```python
from build123d import *

# Parameters (mm, degrees)
SKETCH1_W                = 622.3
SKETCH1_H                = 38.1
BOSS_EXTRUDE1_DEPTH      = 6.35
SKETCH2_R                = 11
CUT_EXTRUDE1_DEPTH       = 1
CUT_EXTRUDE1_DEPTH_BACK  = 7.62
F_0_257_DIAMETER_HOLE2_D = 6.5278


with BuildPart() as part:
    # Sketch1 → Boss-Extrude1 (new body)
    with BuildSketch(Plane(origin=(0, 0, 0), x_dir=(1, 0, 0), z_dir=(0, 1, 0))):
        Rectangle(SKETCH1_W, SKETCH1_H)
    extrude(amount=BOSS_EXTRUDE1_DEPTH)

    # Sketch2 → Cut-Extrude1 (cut, two sides)
    with BuildSketch(Plane(origin=(0, 6.35, 0), x_dir=(1, 0, 0), z_dir=(0, 1, 0))) as cut_extrude1_sk:
        Circle(SKETCH2_R)
    extrude(amount=CUT_EXTRUDE1_DEPTH, mode=Mode.SUBTRACT)
    extrude(cut_extrude1_sk.sketch, amount=-CUT_EXTRUDE1_DEPTH_BACK, mode=Mode.SUBTRACT)

    # F (0.257) Diameter Hole2 (through all)
    with Locations(Plane(origin=(0, 6.35, 0), x_dir=(1, 0, 0), z_dir=(0, 1, 0))):
        with Locations((-279.4, 0), (-241.3, 0)):
            f_0_257_diameter_hole2 = Hole(F_0_257_DIAMETER_HOLE2_D / 2)

    # Mirror1: F (0.257) Diameter Hole2 across plane
    add(f_0_257_diameter_hole2.mirror(Plane(origin=(0, 0, 0), x_dir=(0, 0, 1), z_dir=(1, 0, 0))), mode=Mode.SUBTRACT)


solid = part.part
```
Check sheet for the modelled part. Datum: model origin and axes. Units: mm. Give positions to 0.01 mm unless a question says otherwise; leave off trailing zeros. Order: outer loops, then holes, each group sorted by start corner. A loop starts at its lowest first (then second) coordinate and runs counter-clockwise, first axis right, second up. Notation, with made-up numbers: (84.25, 67.25) -> (121.25, 67.25) arc R9 ccw to (121.25, 76.25) -> close; hole circle Ø6 at (-25, 0.25). An arc over 180 degrees is marked (long way). Use CSV: the item, a comma, the result in double quotes. Start each with the question number.
1) Material ranges on line 1 (Z direction, x = -279.4, y = 3); line 2 (Z direction, x = 0, y = 3.5); line 3 (X direction, y = 2.5, z = -1), recorded low to high. Write a range as from..to.
2) Sectioned sample at B-B, the plane y = 4.75. Record the boundary of the cut face in (x, z).
3) Go/stop test with a flat-tipped pin: P1, Ø5, axis at x = 279.4, z = 0, coming from the +Y side. Record where the tip stops, or that it passes through.
4) Mould release check, pull along X, two halves, no side actions. Record for faces 1 (the face through (-4, 0, -13)), 2 (the face through (-2.38, 3.22, 10.74)): released by +X, released by -X, zero draft, split by the parting line, or undercut.
5) Sectioned sample at A-A, the plane x = 0. Record the boundary of the cut face in (y, z), plus the area to 3 significant figures.
Recorded:
1,line 1,"-19.05..-3.26, 3.26..19.05"
1,line 2,"-19.05..-11, 11..19.05"
1,line 3,"-311.15..-282.51, -276.29..-244.41, -238.19..-10.95, 10.95..238.19, 244.41..276.29, 282.51..311.15"
2,outline,"(-311.15, -19.05) -> (311.15, -19.05) -> (311.15, 19.05) -> (-311.15, 19.05) -> close; hole circle Ø6.53 at (-279.4, 0); hole circle Ø6.53 at (-241.3, 0); hole circle Ø22 at (0, 0); hole circle Ø6.53 at (241.3, 0); hole circle Ø6.53 at (279.4, 0)"
3,P1,"through"
4,face 1,"zero draft"
4,face 2,"undercut"
5,outline,"(0, -19.05) -> (6.35, -19.05) -> (6.35, -11) -> (0, -11) -> close; (0, 11) -> (6.35, 11) -> (6.35, 19.05) -> (0, 19.05) -> close"
5,area,"102 mm2"
